```python
from build123d import *

# Parameters (mm, degrees)
SKETCH_1_W          = 105
SKETCH_1_H          = 100
EXTRUDE_1_DEPTH     = 2
SKETCH_2_W          = 85
SKETCH_2_H          = 60
CUT_EXTRUDE_1_DEPTH = 2
SKETCH_4_R          = 1
EXTRUDE_2_DEPTH     = 10
SKETCH_5_W          = 105
SKETCH_5_H          = 10
CUT_EXTRUDE_2_DEPTH = 10
SKETCH_7_R          = 0.5
EXTRUDE_3_DEPTH     = 6.4724949
SKETCH_8_R          = 0.5
EXTRUDE_4_DEPTH     = 85


with BuildPart() as part:
    # 스케치1 → 보스-돌출1 (new body)
    with BuildSketch(Plane(origin=(0, 0, 0), x_dir=(1, 0, 0), z_dir=(0, 1, 0))):
        Rectangle(SKETCH_1_W, SKETCH_1_H)
    extrude(amount=EXTRUDE_1_DEPTH)

    # 스케치2 → 컷-돌출1 (cut)
    with BuildSketch(Plane(origin=(0, 2, 0), x_dir=(1, 0, 0), z_dir=(0, 1, 0))):
        with Locations((0, -20)):
            Rectangle(SKETCH_2_W, SKETCH_2_H)
    extrude(amount=-CUT_EXTRUDE_1_DEPTH, mode=Mode.SUBTRACT)

    # 스케치4 → 보스-돌출2 (add)
    with BuildSketch(Plane(origin=(0, 2, 0), x_dir=(1, 0, 0), z_dir=(0, 1, 0))):
        with Locations(Location((45.5, -36, 0), (0, 0, 270))):
            Circle(SKETCH_4_R)
        with Locations(Location((-47.5, -36, 0), (0, 0, 270))):
            Circle(SKETCH_4_R)
    extrude(amount=EXTRUDE_2_DEPTH)

    # 스케치5 → 컷-돌출2 (cut)
    with BuildSketch(Plane(origin=(0, 2, 0), x_dir=(1, 0, 0), z_dir=(0, 1, 0))):
        with Locations((0, 45)):
            Rectangle(SKETCH_5_W, SKETCH_5_H)
    extrude(amount=-CUT_EXTRUDE_2_DEPTH, mode=Mode.SUBTRACT)

    # 스케치7 → 보스-돌출3 (add)
    with BuildSketch(Plane(origin=(52.5, 0, 0), x_dir=(0, 0, -1), z_dir=(1, 0, 0))):
        with Locations(Location((-47.972067637, 1, 0), (0, 0, 180))):
            Circle(SKETCH_7_R)
        with Locations(Location((-27.972067637, 1, 0), (0, 0, 180))):
            Circle(SKETCH_7_R)
        with Locations(Location((-7.972067637, 1, 0), (0, 0, 180))):
            Circle(SKETCH_7_R)
        with Locations(Location((12.027932363, 1, 0), (0, 0, 180))):
            Circle(SKETCH_7_R)
        with Locations(Location((32.027932363, 1, 0), (0, 0, 180))):
            Circle(SKETCH_7_R)
    extrude(amount=EXTRUDE_3_DEPTH)

    # 스케치8 → 보스-돌출4 (add)
    with BuildSketch(Plane(origin=(-42.5, 0, 0), x_dir=(0, 0, -1), z_dir=(1, 0, 0))):
        with Locations((-46.082216043, 0.875077013)):
            Circle(SKETCH_8_R)
        with Locations((-21.082216043, 0.875077013)):
            Circle(SKETCH_8_R)
        with Locations((3.917783957, 0.875077013)):
            Circle(SKETCH_8_R)
    extrude(amount=EXTRUDE_4_DEPTH)


solid = part.part
```
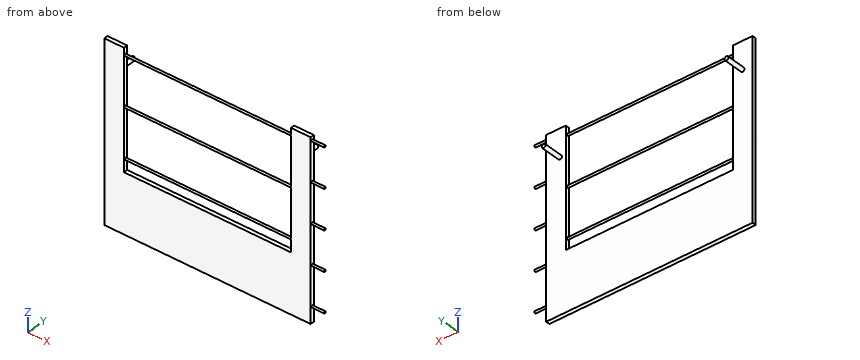
Geometry: final body of the model. Coordinates: model frame, mm. Round coordinates to 2 decimals unless told otherwise and drop trailing zeros. Order: outer loops, then holes, each group sorted by start corner. A loop starts at its lowest first (then second) coordinate and runs counter-clockwise, first axis right, second up. Notation, with made-up numbers: M 27.5,-13 L 40.5,-13 A12 cw 40.5,-9 Z; hole C -3.5,-31 d5. An arc over 180 degrees is marked long. Use one line per item in the form item = value. Start each with the question number.
Q1. Pin query (flat end, axial travel): pin 1 Ø0.6 at (x, y) = (-7, 1.5) entering from +Z; pin 2 Ø8 at (x, z) = (32, 15.5) entering from +Y; pin 3 Ø10 at (x, z) = (37, 1) entering from -Y; pin 4 Ø0.6 at (y, z) = (0.5, 33) entering from +X. Return the tip coordinate at first contact, or that it passes through.
Q2. Cut plane C-C (x = -23). Return loops of the section in (y, z), and give its area (3 significant figures).
Q3. Cut plane A-A (z = 17.5). Return loops of the section in (x, y), and give its area (3 significant figures).
Q4. Cut plane B-B (y = 4.25). Return loops of the section in (x, z).
Q5. Cut plane D-D (x = 48). Return loops of the section in (y, z).
Q6. Material intervals for line 1 (X direction, y = 1.25, z = 23.5); line 2 (Y direction, x = 47, z = 44.5); line 3 (Z direction, x = 38.5, y = 1.75), sorted ascending. Write a range as [from, to].
Geometry results:
q1.pin_1 = 46.46
q1.pin_2 = through
q1.pin_3 = 0.38
q1.pin_4 = 52.5
q2.outline = M 0,-40 L 2,-40 L 2,-10 L 0,-10 Z; C 0.88,-3.92 d1; C 0.88,21.08 d1; C 0.88,46.08 d1
q2.area = 62.4 mm^2
q3.outline = M -52.5,0 L -42.5,0 L -42.5,2 L -52.5,2 Z; M 42.5,0 L 52.5,0 L 52.5,2 L 42.5,2 Z
q3.area = 40.0 mm^2
q4.outline = C -47.5,36 d2; C 45.5,36 d2
q5.outline = M 0,-40 L 2,-40 L 2,50 L 0,50 Z
q6.line_1 = [-52.5, -42.5], [42.5, 52.5]
q6.line_2 = [0, 2]
q6.line_3 = [-40, -10]
